from build123d import *

# Parameters (mm, degrees)
SKETCH1_W           = 22.4
SKETCH1_H           = 22.9
BOSS_EXTRUDE1_DEPTH = 2
SKETCH2_R           = 1
CUT_EXTRUDE1_DEPTH  = 5
SKETCH4_R           = 3.9
BOSS_EXTRUDE3_DEPTH = 5


with BuildPart() as part:
    # Sketch1 → Boss-Extrude1 (new body)
    with BuildSketch(Plane.XY):
        Rectangle(SKETCH1_W, SKETCH1_H)
    extrude(amount=BOSS_EXTRUDE1_DEPTH)

    # Sketch2 → Cut-Extrude1 (cut)
    with BuildSketch(Plane.XY.offset(2)):
        with Locations((-8.7, 0)):
            Circle(SKETCH2_R)
        with Locations((8.7, 0)):
            Circle(SKETCH2_R)
        with Locations((8.7, 6)):
            Circle(SKETCH2_R)
    extrude(amount=-CUT_EXTRUDE1_DEPTH, mode=Mode.SUBTRACT)

    # Sketch4 → Boss-Extrude3 (add)
    with BuildSketch(Plane(origin=(0, 0, 0), x_dir=(-1, 0, 0), z_dir=(0, 0, -1))):
        with Locations((0, 5.25)):
            Circle(SKETCH4_R)
    extrude(amount=BOSS_EXTRUDE3_DEPTH)


solid = part.part
Build history of the part. All positions in model axes, mm. A direction names the side the tool comes from. Give positions to 0.01 mm unless a question says otherwise; leave off trailing zeros. Order: outer loops, then holes, each group sorted by start corner. A loop starts at its lowest first (then second) coordinate and runs counter-clockwise, first axis right, second up. Notation, with made-up numbers: M 67,10 L 108,10 A28 ccw 108,38 Z; hole C 38,76.25 d11. An arc over 180 degrees is marked long. Use one line per item in the form item = value.
1) Saw through at C-C (y = 0). Give the cut face in (x, z).
Calculated:
outline = M -11.2,0 L -9.7,0 L -9.7,2 L -11.2,2 Z; M -7.7,0 L 7.7,0 L 7.7,2 L -7.7,2 Z; M 9.7,0 L 11.2,0 L 11.2,2 L 9.7,2 Z
2) Tool access for faces 1 (the face through (2.87, 7.89, -2.46)), 2 (the face through (0, 0, 2)): list every direction of +Z, -Z, +X, -X, +Y, -Y with a clear straight run to the whole face (end or side of a thin tool).
Calculated:
face_1 = -Z
face_2 = +Z, +X, -X, +Y, -Y
3) Saw through at D-D (y = 6). Give the cut face in (x, z), plus the area to 3 significant figures.
Calculated:
outline = M -11.2,0 L -3.83,0 L -3.83,-5 L 3.83,-5 L 3.83,0 L 7.7,0 L 7.7,2 L -11.2,2 Z; M 9.7,0 L 11.2,0 L 11.2,2 L 9.7,2 Z
area = 79.1 mm2
4) Saw through at B-B (z = 0.5). Give the cut face in (x, y), plus the area to 3 significant figures.
Calculated:
outline = M -11.2,-11.45 L 11.2,-11.45 L 11.2,11.45 L -11.2,11.45 Z; hole C -8.7,0 d2; hole C 8.7,0 d2; hole C 8.7,6 d2
area = 504 mm2
5) Saw through at A-A (x = -8.7). Give the cut face in (y, z), plus the area to 3 significant figures.
Calculated:
outline = M -11.45,0 L -1,0 L -1,2 L -11.45,2 Z; M 1,0 L 11.45,0 L 11.45,2 L 1,2 Z
area = 41.8 mm2
6) Probe probe 1 along Y at (x, z) = (8.7, 0.6); probe 2 along Y at (x, z) = (-8.7, 1.2); probe 3 along Y at (x, z) = (8.25, 0.75). List the from-to ranges inside material, lowest first.
Calculated:
probe_1 = -11.45 to -1, 1 to 5, 7 to 11.45
probe_2 = -11.45 to -1, 1 to 11.45
probe_3 = -11.45 to -0.89, 0.89 to 5.11, 6.89 to 11.45
7) Drop a flat-ended pin along its axis: pin 1 (3 mm diameter, centred on x = -2, y = -7.5, fed in from -Z). Give the stop position or say it passes through.
Calculated:
pin_1 = 0
8) Two-plate mould, pull along Y, no slides. Class faces 3 (the face through (9.654, 0.3, 1.014)), 4 (the face through (0, -11.45, 1)), 5 (the face through (0, 5, -5)): released by +Y, released by -Y, zero draft, split by the parting line, or undercut.
Calculated:
face_3 = undercut
face_4 = released by -Y
face_5 = zero draft
